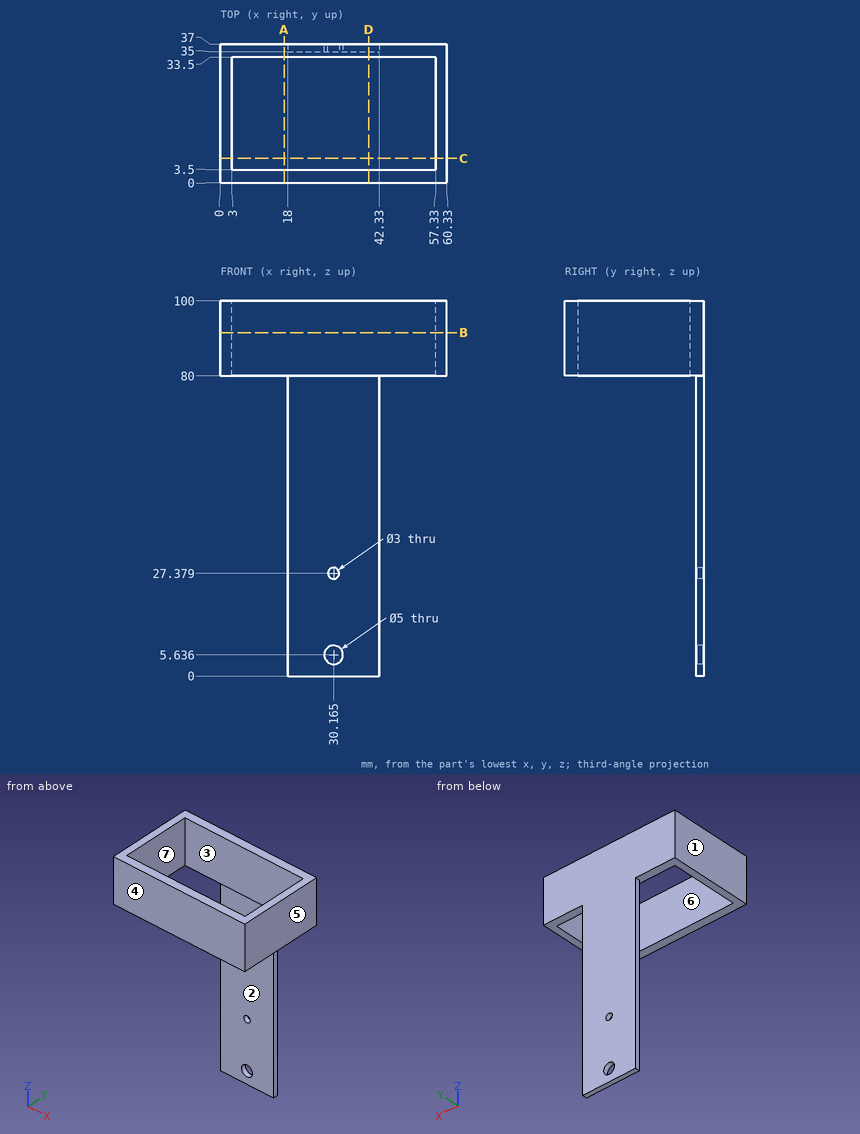
Geometry: see drawing. Coordinates: mm, zero at the bounding-box minimum. A direction names the side the tool comes from. Coordinates: 2 decimals unless noted, no trailing zeros. Write each loop counter-clockwise with the first axis right and the second up, starting at its lowest first coordinate (ties: lowest second). Pieces come first, ordered by that corner, then holes.
1) Set-up query: the marked faces 1, 2 and 3. Return all of +Z, -Z, +X, -X, +Y, -Y with unobstructed straight access to the full face (end or side cutting, diameter ignored); none if empty.
2) Material intervals for line 1 along X through (y, z) = (4.5, 82); line 2 along Z through (x, y) = (57.5, 20); line 3 along Y through (x, z) = (35, 34), sorted ascending.
3) Mould query, pull axis X, two halves, no side actions, for the marked faces 4, 5, 6 and 7. Classes: pulls with the +X half, pulls with the -X half, needs draft (parallel to the pull), parting line crosses it, or undercut.
4) Section A-A on x = 17. Output: boundary loops of the cut face in (y, z).
5) Section B-B on z = 91.5. Output: boundary loops of the cut face in (x, y).
6) Section D-D on x = 39.5. Output: boundary loops of the cut face in (y, z).
7) Pin query (flat end, axial travel): pin 1 Ø5 at (x, z) = (18, 60) entering from -Y; pin 2 Ø16 at (x, z) = (38, 93.5) entering from -Y; pin 3 Ø1.6 at (y, z) = (36, 51) entering from +X; pin 4 Ø1 at (y, z) = (36.5, 58.5) entering from -X. Return the tip coordinate at first contact, or that it passes through.
8) Section C-C on y = 6.5. Output: boundary loops of the cut face in (x, z), and give its area (3 significant figures).
Check result:
1. face 1: +Z, -Z, -X, +Y, -Y
1. face 2: -Z, +X, -X, -Y
1. face 3: +Z, -Z
2. line 1: x = 0 to 3, 57.33 to 60.33
2. line 2: z = 80 to 100
2. line 3: y = 35 to 37
3. face 4: needs draft
3. face 5: pulls with the +X half
3. face 6: undercut
3. face 7: undercut
4. outline: (0, 80) - (3.5, 80) - (3.5, 100) - (0, 100) - close; (33.5, 80) - (37, 80) - (37, 100) - (33.5, 100) - close
5. outline: (0, 0) - (60.33, 0) - (60.33, 37) - (0, 37) - close; hole (3, 3.5) - (57.33, 3.5) - (57.33, 33.5) - (3, 33.5) - close
6. outline: (0, 80) - (3.5, 80) - (3.5, 100) - (0, 100) - close; (33.5, 80) - (35, 80) - (35, 0) - (37, 0) - (37, 100) - (33.5, 100) - close
7. pin 1: stops at y = 35
7. pin 2: stops at y = 0
7. pin 3: stops at x = 42.33
7. pin 4: stops at x = 18
8. outline: (0, 80) - (3, 80) - (3, 100) - (0, 100) - close; (57.33, 80) - (60.33, 80) - (60.33, 100) - (57.33, 100) - close
8. area: 120 mm2
